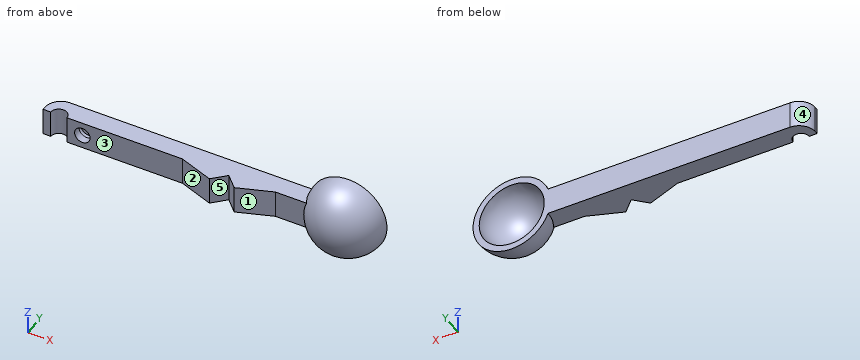
from build123d import *

# Parameters (mm, degrees)
SKETCH1_W               = 107.95
SKETCH1_H               = 11.1125
BOSS_EXTRUDE1_DEPTH     = 7.9375
CUT_EXTRUDE1_DEPTH      = 1
CUT_EXTRUDE1_DEPTH_BACK = 12.1125
BOSS_EXTRUDE2_DEPTH     = 11.1125
FILLET1_R               = 6.604
REVOLVE1_ANGLE          = 180


with BuildPart() as part:
    # Sketch1 → Boss-Extrude1 (new body)
    with BuildSketch(Plane(origin=(0, 0, 0), x_dir=(1, 0, 0), z_dir=(0, 1, 0))):
        with Locations((53.975, 5.55625)):
            Rectangle(SKETCH1_W, SKETCH1_H)
    extrude(amount=BOSS_EXTRUDE1_DEPTH)

    # Sketch2 → Cut-Extrude1 (cut, two sides)
    with BuildSketch(Plane.XY) as cut_extrude1_sk:
        with BuildLine():
            Line((3.175, 0), (9.779, 0))
            ThreePointArc((9.779, 0), (6.477, 3.302), (3.175, 0))
        make_face()
    extrude(amount=CUT_EXTRUDE1_DEPTH, mode=Mode.SUBTRACT)
    extrude(cut_extrude1_sk.sketch, amount=-CUT_EXTRUDE1_DEPTH_BACK, mode=Mode.SUBTRACT)

    # Sketch2<4> → Boss-Extrude2 (add, through all)
    with BuildSketch(Plane.XY):
        Polygon((76.2, 0), (57.15, 0), (71.12, -5.08), align=None)
        Polygon((95.25, 0), (76.2, 0), (81.28, -5.08), align=None)
    extrude(amount=-BOSS_EXTRUDE2_DEPTH)

    # Fillet1
    fillet1_edges = [part.edges().sort_by_distance(p)[0] for p in [
        (0, 7.9375, -5.55625),
    ]]
    fillet(fillet1_edges, radius=FILLET1_R)

    # Sketch3 → Revolve1 (revolve)
    with BuildSketch(Plane(origin=(0, 7.9375, 0), x_dir=(1, 0, 0), z_dir=(0, 1, 0))):
        with BuildLine():
            Line((104.775, 5.55625), (136.525, 5.55625))
            ThreePointArc((136.525, 5.55625), (120.65, -10.31875), (104.775, 5.55625))
        make_face()
    revolve(axis=Axis((104.775, 7.9375, -5.55625), (1, 0, 0)), revolution_arc=REVOLVE1_ANGLE)

    # Sketch5 → Cut-Revolve2 (revolve, cut)
    with BuildSketch(Plane(origin=(0, 7.9375, 0), x_dir=(1, 0, 0), z_dir=(0, 1, 0))):
        with BuildLine():
            Line((107.315, 5.55625), (133.985, 5.55625))
            ThreePointArc((133.985, 5.55625), (120.65, -7.77875), (107.315, 5.55625))
        make_face()
    revolve(axis=Axis((107.315, 7.9375, -5.55625), (1, 0, 0)), mode=Mode.SUBTRACT)

    # Sketch6 → Cut-Revolve3 (revolve, cut)
    with BuildSketch(Plane.XY.offset(-5.55625)):
        Polygon((16.129, 0), (19.304, 0), (19.304, 3.175), (19.685, 3.175), (19.685, 4.953), (16.129, 4.953), (16.129, 3.175), align=None)
    revolve(axis=Axis((16.129, 0, -5.55625), (0, 1, 0)), mode=Mode.SUBTRACT)


solid = part.part
Here's how the part is built. I have some questions about the finished solid (model axes, mm). Face numbers are marked on the shaded views. A direction names the side the tool comes from. Round coordinates to 2 decimals unless told otherwise and drop trailing zeros. Order: outer loops, then holes, each group sorted by start corner. A loop starts at its lowest first (then second) coordinate and runs counter-clockwise, first axis right, second up. Notation, with made-up numbers: M 43,32 L 61,32 A14 cw 61,58 Z; hole C 5.5,27.25 d4. An arc over 180 degrees is marked long. Return JSON: item names as keys, results as strings. Group by question number.
1. If we section it at A-A on y = -1.5: State how many separate pieces and enclosed holes the cut face has, then the cut area to 3 significant figures.
2. Please list where these lines run through material, in increasing order: probe 1 along Z at (x, y) = (97, 4.75); probe 2 along Y at (x, z) = (30, -8); probe 3 along X at (y, z) = (1.25, -6).
3. On a 3-axis mill with a long thin cutter (end or side, diameter ignored), from which of +Z, -Z, +X, -X, +Y, -Y can I reach the whole of each face in a straight line? I mean the marked faces 1 and 2. Say none if no direction works.
4. If we section it at B-B on x = 43: List the corners of the cut face in (y, z) for me.
5. If we section it at C-C on y = 6.25: List the corners of the cut face in (x, z) for me.
6. If we section it at D-D on z = 6.5: List the corners of the cut face in (x, y) for me.
7. I'm going to push flat-ended pins straight in: pin 1 Ø2 at (y, z) = (2, 2.5) entering from +X; pin 2 Ø3 at (x, y) = (115, -3) entering from +Z; pin 3 Ø4 at (x, y) = (89, 2.5) entering from -Z. Where does each tip first touch, or does it pass through?
8. If we mould it in two halves opening along X, with no side actions, what happens to the marked faces 3, 4 and 5? For each: pulls with the +X half, pulls with the -X half, needs draft (parallel to the pull), parting line crosses it, or undercut.
Reply:
{
 "1": {"separate pieces": "3", "enclosed holes": "1", "area": "531 mm^2"},
 "2": {"probe 1": "-11.11 to 0", "probe 2": "0 to 7.94", "probe 3": "0 to 3.42, 9.53 to 12.99, 19.27 to 109.12, 132.18 to 135.04"},
 "3": {"face 1": "+Z, -Z, -Y", "face 2": "+Z, -Z, -X, -Y"},
 "4": {"outline": "M 0,-11.11 L 7.94,-11.11 L 7.94,0 L 0,0 Z"},
 "5": {"outline": "M 2.19,-11.11 L 105.88,-11.11 A15.79 ccw long 105.88,0 L 2.19,0 Z; hole C 120.65,-5.56 d26.46"},
 "6": {"outline": "M 110.32,7.94 A10.33 ccw 130.98,7.94 L 126.35,7.94 A5.7 cw 114.95,7.94 Z"},
 "7": {"pin 1": "x = 133.72", "pin 2": "z = 6.07", "pin 3": "z = -11.11"},
 "8": {"face 3": "needs draft", "face 4": "pulls with the -X half", "face 5": "undercut"}
}
